Could you check a few things on this model? Use its own coordinates, in mm. Face numbers are marked on the shaded views. A direction names the side the tool comes from. Give positions to 0.01 mm unless a question says otherwise; leave off trailing zeros. Write each loop counter-clockwise with the first axis right and the second up, starting at its lowest first coordinate (ties: lowest second). Pieces come first, ordered by that corner, then holes. Notation, with made-up numbers: (0.5, 29) - (53.5, 29) arc R26 cw to (53.5, 59) - close; hole circle Ø5 at (34, 6). An arc over 180 degrees is marked (long way). Answer as CSV lines item,"result". Start each with the question number.
Q1. We'd pull the mould along X, two halves only. Please class the marked faces 3, 4, 5 and 6: pulls with the +X half, pulls with the -X half, needs draft (parallel to the pull), parting line crosses it, or undercut.
Q2. If I drill on line 1 along Z through (x, y) = (5, 0.3); line 2 along X through (y, z) = (1.65, 5.25); line 3 along Y through (x, z) = (5.75, 2.25), over which ranges is the centre line in solid material (lowest first)?
Q3. Will this pin go through, and if not, where does the flat tip stop? pin 1 Ø4 at (x, z) = (6, 5) entering from -Y.
Q4. On a 3-axis mill with a long thin cutter (end or side, diameter ignored), from which of +Z, -Z, +X, -X, +Y, -Y can I reach the whole of each face in a straight line? I mean the marked faces 1 and 2. Say none if no direction works.
Q5. Imagine slicing it at B-B on x = 7. List the corners of the cut face in (y, z) for me, and give its area (3 significant figures).
Q6. Imagine slicing it at A-A on y = 1.9. List the corners of the cut face in (x, z) for me, and give its area (3 significant figures).
Q7. Imagine slicing it at C-C on z = 6.5. List the corners of the cut face in (x, y) for me.
```python
from build123d import *

# Parameters (mm, degrees)
MAINBASESKETCH_W         = 7.9
MAINBASESKETCH_H         = 3.2
MAINBASEEXTRUDE_DEPTH    = 7.9
MAINBASESHELL_T          = -1.2
SKETCH171_W              = 5.5
SKETCH171_H              = 1.191135725
BOSS_EXTRUDE23_DEPTH     = 2
CUT_EXTRUDE58_DEPTH      = 12.83470157
CUT_EXTRUDE58_DEPTH_BACK = 12.83470157


with BuildPart() as part:
    # MainBaseSketch → MainBaseExtrude (new, symmetric)
    with BuildSketch(Plane.XY):
        with Locations((4.631967213, 1.6)):
            Rectangle(MAINBASESKETCH_W, MAINBASESKETCH_H)
    extrude(amount=MAINBASEEXTRUDE_DEPTH, both=True)

    # MainBaseShell
    mainbaseshell_openings = [part.faces().sort_by_distance(p)[0] for p in [
        (4.631967213, 0, 0),
    ]]
    offset(amount=MAINBASESHELL_T, openings=mainbaseshell_openings, kind=Kind.INTERSECTION)

    # Sketch171 → Boss-Extrude23 (add)
    with BuildSketch(Plane(origin=(0, 2, 0), x_dir=(-1, 0, 0), z_dir=(0, -1, 0))):
        with Locations((-4.631967213, -0.595567863)):
            Rectangle(SKETCH171_W, SKETCH171_H)
    extrude(amount=BOSS_EXTRUDE23_DEPTH)

    # Sketch173 → Cut-Extrude58 (cut, two sides: drawn at the far end of the back side and taken through both)
    with BuildSketch(Plane(origin=(0, 2, 0), x_dir=(-1, 0, 0), z_dir=(0, -1, 0)).offset(-CUT_EXTRUDE58_DEPTH_BACK)):
        Polygon((-7.381967213, 0), (-8.581967213, 0), (-8.581967213, 7.9), (-0.681967213, 7.9), (-0.681967213, 0), align=None)
    extrude(amount=CUT_EXTRUDE58_DEPTH + CUT_EXTRUDE58_DEPTH_BACK, mode=Mode.SUBTRACT)


solid = part.part
```
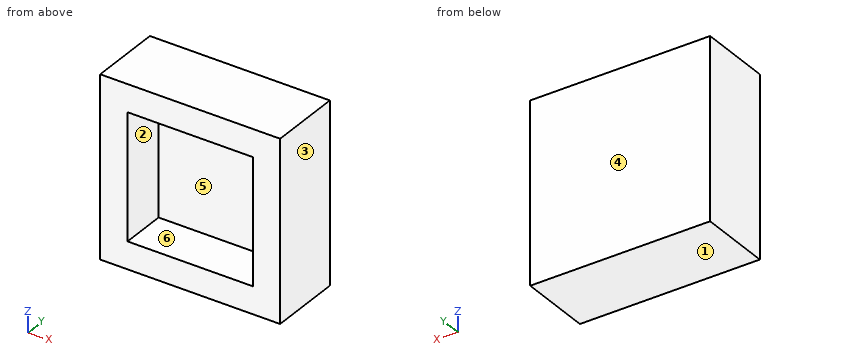
Conclusion:
1,face 3,"pulls with the +X half"
1,face 4,"needs draft"
1,face 5,"undercut"
1,face 6,"undercut"
2,line 1,"0 to 1.19, 6.7 to 7.9"
2,line 2,"0.68 to 1.88, 7.38 to 8.58"
2,line 3,"2 to 3.2"
3,pin 1,"y = 0"
4,face 1,"-Z, +X, -X, +Y, -Y"
4,face 2,"-Y"
5,outline,"(0, 0) - (3.2, 0) - (3.2, 7.9) - (0, 7.9) - (0, 6.7) - (2, 6.7) - (2, 1.19) - (0, 1.19) - close"
5,area,"14.3 mm^2"
6,outline,"(0.68, 0) - (8.58, 0) - (8.58, 7.9) - (0.68, 7.9) - close; hole (1.88, 1.19) - (7.38, 1.19) - (7.38, 6.7) - (1.88, 6.7) - close"
6,area,"32.1 mm^2"
7,outline,"(0.68, 0) - (1.88, 0) - (1.88, 2) - (7.38, 2) - (7.38, 0) - (8.58, 0) - (8.58, 3.2) - (0.68, 3.2) - close"
